Autodesk Inventor part; units mm, degrees
ref_plane "YZ Plane" through (0, 0, 0) normal (1, 0, 0) x (0, 1, 0)
ref_plane "XZ Plane" through (0, 0, 0) normal (0, 1, 0) x (-1, 0, 0)
ref_plane "XY Plane" through (0, 0, 0) normal (0, 0, 1) x (1, 0, 0)
sketch "スケッチ1" plane through (0, 0, 0) normal (0, 1, 0) x (-1, 0, 0)
  line L0 (0, 0) -> (45, 0)
  line L1 (45, 0) -> (45, -15)
  line L2 (0, -40) -> (0, 0)
  line L3 (45, 0) -> (45, -15)
  line L4 (45, 0) -> (60, 0) construction
  line L5 (0, -40) -> (15, -40)
  line L6 (0, -40) -> (15, -40) construction
  line L7 (15, -40) -> (45, -15)
  line L8 (15, -40) -> (0, -40)
  dimension "d2" = 15
  dimension "d3" = 90
  dimension "d4" = 15
  dimension "d5" = 0
extrude "押し出し1" add sketch "スケッチ1" along normal blind 3
sketch "スケッチ2" plane through (0, 3, 0) normal (0, 1, 0) x (1, 0, 0)
  line L0 (-45, 0) -> (0, 0)
  line L1 (-45, 15) -> (-45, 0)
  line L2 (0, 0) -> (0, 40)
  line L3 (0, 40) -> (-15, 40)
  point P0 (-36, 7.5)
  point P1 (-7.5, 30)
  point P2 (-29, 7.5)
  point P3 (-22, 7.5)
  point P4 (-7.5, 20)
  point P5 (-7.5, 10)
  dimension "d8" = 7.5
  dimension "d9" = 9
  dimension "d10" = 7
  dimension "d11" = 7
  dimension "d12" = 7.5
  dimension "d13" = 7.5
  dimension "d14" = 7.5
  dimension "d15" = 10
  dimension "d16" = 10
  dimension "d17" = 10
  dimension "d18" = 7.5
  dimension "d19" = 7.5
hole "穴1" at (-36, 3, -7.5) at (-7.5, 3, -30) at (-29, 3, -7.5) at (-22, 3, -7.5) at (-7.5, 3, -20) at (-7.5, 3, -10) direction (0, -1, 0) diameter 3.2 end through all
fillet "フィレット1" radius 2 5 edges at (0, 1.5, -40) (0, 1.5, 0) (-45, 1.5, 0) (-45, 1.5, -15) (-15, 1.5, -40)
properties part number "射出_固定3" material "アルミニウム 6061"
The listing builds one solid part. Answer for the finished solid, in the listing's coordinates (mm). Coordinates: 2 decimals unless noted, no trailing zeros. Loops run counter-clockwise (first coordinate to the right, second up) from the corner with the lowest first, then second, coordinate; pieces in that order, holes last. Notation, with made-up numbers: (7, -24.75) -> (47, -24.75) arc R35 cw to (47, 13.25) -> close; hole circle Ø1 at (71, 38). An arc over 180 degrees is marked (long way). Write item = value, one per line. Start each with the question number.
1) A cutting plane is placed at B-B (x = -7.5). Give the vertices of the cut face in (y, z), then the cut area to 3 significant figures.
2) A cutting plane is placed at A-A (z = -20). Give the vertices of the cut face in (x, y).
3) The mould has two halves that part along X. Classify faces 1 (the face through (-29.717, 1.479, -27.736)), 2 (the face through (-17, 3, -15)), 3 (the face through (-5.94, 1.48, -20.35)): released by +X, released by -X, zero draft, split by the parting line, or undercut.
4) A cutting plane is placed at D-D (x = -36). Give the vertices of the cut face in (y, z), then the cut area to 3 significant figures.
5) Given pin 1 Ø3 at (x, z) = (-36, -7.5) entering from -Y; pin 2 Ø5 at (x, z) = (-29, -7.5) entering from +Y; pin 3 Ø1.5 at (y, z) = (1.5, -26.5) entering from -X, each flat-ended and moving along its own axis, determine where each tip first touches the part or whether it passes through.
6) Straight lines are drawn through the part: line 1 (Z direction, x = -7.5, y = 2.2); line 2 (X direction, y = 0.85, z = -7.5); line 3 (X direction, y = 0.1, z = -10). For each, find the intervals that lie inside material, in ascending order. Write a range as from..to.
7) A cutting plane is placed at C-C (z = -7.5). Give the vertices of the cut face in (x, y), then the cut area to 3 significant figures.
Responses:
q1.outline = (0, -40) -> (3, -40) -> (3, -31.6) -> (0, -31.6) -> close; (0, -28.4) -> (3, -28.4) -> (3, -21.6) -> (0, -21.6) -> close; (0, -18.4) -> (3, -18.4) -> (3, -11.6) -> (0, -11.6) -> close; (0, -8.4) -> (3, -8.4) -> (3, 0) -> (0, 0) -> close
q1.area = 91.2 mm²
q2.outline = (-39, 0) -> (-9.1, 0) -> (-9.1, 3) -> (-39, 3) -> close; (-5.9, 0) -> (0, 0) -> (0, 3) -> (-5.9, 3) -> close
q3.face_1 = released by -X
q3.face_2 = zero draft
q3.face_3 = undercut
q4.outline = (0, -22.5) -> (3, -22.5) -> (3, -9.1) -> (0, -9.1) -> close; (0, -5.9) -> (3, -5.9) -> (3, 0) -> (0, 0) -> close
q4.area = 57.9 mm²
q5.pin_1 = through
q5.pin_2 = 3
q5.pin_3 = -32.1
q6.line_1 = -40..-31.6, -28.4..-21.6, -18.4..-11.6, -8.4..0
q6.line_2 = -45..-37.6, -34.4..-30.6, -27.4..-23.6, -20.4..0
q6.line_3 = -45..-9.1, -5.9..0
q7.outline = (-45, 0) -> (-37.6, 0) -> (-37.6, 3) -> (-45, 3) -> close; (-34.4, 0) -> (-30.6, 0) -> (-30.6, 3) -> (-34.4, 3) -> close; (-27.4, 0) -> (-23.6, 0) -> (-23.6, 3) -> (-27.4, 3) -> close; (-20.4, 0) -> (0, 0) -> (0, 3) -> (-20.4, 3) -> close
q7.area = 106 mm²
